Here's how the part is built. I have some questions about the finished solid (model axes, mm). A direction names the side the tool comes from. Give positions to 0.01 mm unless a question says otherwise; leave off trailing zeros. Write each loop counter-clockwise with the first axis right and the second up, starting at its lowest first coordinate (ties: lowest second). Pieces come first, ordered by that corner, then holes. Notation, with made-up numbers: (-22, 16.25) - (18, 16.25) arc R19 ccw to (18, 48.25) - close; hole circle Ø6 at (14.5, 57.25). An arc over 180 degrees is marked (long way). Write each question's results on one line, items separated by ' | '. Start each with the question number.
Item 1: Suppose I cut it at A-A on y = 18. Count the separate pieces of the cut face and the enclosed holes in it, then the cut area to 3 significant figures.
Item 2: Suppose I cut it at C-C on x = -25. List the corners of the cut face in (y, z) for me.
Item 3: Which directions (+Z, -Z, +X, -X, +Y, -Y) give clear straight access to the entire face, cutting with the end or side of a thin tool? Please do faces 1 (the flat face through (-50, -18, -18)), 2 (the flat face through (-39, -14, -28)), 3 (the flat face through (-3, 0, -16)).
Item 4: We'd pull the mould along Z, two halves only. Please class faces 4 (the flat face through (-28, 14, -26)), 5 (the flat face through (-1, 24, -1)), 6 (the cylindrical face through (-1.175, 2.494, -11.034)): +Z half, -Z half, draft (parallel to the pull), parting line (faces both ways), or undercut.
Item 5: Will these pins go through, and if not, where does the flat tip stop? P1, Ø3, axis at x = -55, y = 18, coming from the -Z side; P2, Ø5, axis at x = -79.5, y = -15.5, coming from the +Z side; P3, Ø2.5, axis at x = -43, y = -19, coming from the -Z side; P4, Ø4, axis at y = -18.5, z = -27, coming from the -X side.
Item 6: Suppose I cut it at B-B on y = 0. List the corners of the cut face in (x, z) for me.
Item 7: Suppose I cut it at D-D on z = -31. List the corners of the cut face in (x, y) for me, then the cut area to 3 significant figures.
Item 8: Please list where these lines run through material, in increasing order: line 1 along Y through (x, z) = (-24, -23.5); line 2 along Z through (x, y) = (-0.35, 0); line 3 along X through (y, z) = (-3, -6.5).
```python
from build123d import *

# Parameters (mm, degrees)
PAD_DEPTH         = 40
PAD001_DEPTH      = 25
POCKET_DEPTH      = 25.001
POCKET_DEPTH_BACK = -25.001
POCKET001_DEPTH   = 93
SKETCH003_R       = 1.7
POCKET002_DEPTH   = 40.001
SKETCH005_R       = 2.7
POCKET003_DEPTH   = 96.601
CHAMFER_SIZE      = 2
FILLET_R          = 1


with BuildPart() as part:
    # Sketch → Pad (new body)
    with BuildSketch(Plane.XY):
        Polygon((0, 25), (-96, 25), (-96, 11), (-3, 11), (-3, -11), (-96, -11), (-96, -25), (0, -25), align=None)
    extrude(amount=-PAD_DEPTH)

    # Sketch004 → Pad001 (join, symmetric)
    with BuildSketch(Plane.XZ):
        Polygon((0, -7), (0, -13), (0.6, -12.4), (0.6, -7.6), align=None)
        Polygon((0, -27), (0, -33), (0.6, -32.4), (0.6, -27.6), align=None)
    extrude(amount=PAD001_DEPTH, both=True)

    # Sketch001 → Pocket (cut, two sides)
    with BuildSketch(Plane.XZ) as pocket_sk:
        Polygon((-3, -40), (-96, -21), (-96, -18), (-3, -18), (-3, 0), (-97, 0), (-97, -40), align=None)
    extrude(amount=-POCKET_DEPTH, mode=Mode.SUBTRACT)
    extrude(pocket_sk.sketch, amount=-POCKET_DEPTH_BACK, mode=Mode.SUBTRACT)

    # Sketch002 → Pocket001 (cut)
    with BuildSketch(Plane.YZ.offset(-3)):
        Polygon((-22, -41), (-22, -21), (-14, -21), (-14, -40), (14, -40), (14, -21), (22, -21), (22, -41), align=None)
    extrude(amount=-POCKET001_DEPTH, mode=Mode.SUBTRACT)

    # Sketch003 → Pocket002 (cut, through all)
    with BuildSketch(Plane.XY):
        with Locations((-85, 18)):
            Circle(SKETCH003_R)
        with Locations((-25, 18)):
            Circle(SKETCH003_R)
        with Locations((-25, -18)):
            Circle(SKETCH003_R)
        with Locations((-85, -18)):
            Circle(SKETCH003_R)
        with Locations((-55, -18)):
            Circle(SKETCH003_R)
        with Locations((-55, 18)):
            Circle(SKETCH003_R)
    extrude(amount=-POCKET002_DEPTH, mode=Mode.SUBTRACT)

    # Sketch005 → Pocket003 (cut, through all)
    with BuildSketch(Plane.YZ.offset(0.6)):
        with Locations((0, -10)):
            Circle(SKETCH005_R)
        with Locations((0, -30)):
            Circle(SKETCH005_R)
    extrude(amount=-POCKET003_DEPTH, mode=Mode.SUBTRACT)

    # Chamfer
    chamfer_edges = [part.edges().sort_by_distance(p)[0] for p in [
        (-1.5, 25, 0),
        (-1.5, -25, 0),
    ]]
    chamfer(chamfer_edges, length=CHAMFER_SIZE)

    # Fillet
    fillet_edges = [part.edges().sort_by_distance(p)[0] for p in [
        (0, 0, 0),
        (0, 0, -40),
        (-3, 0, 0),
        (-3, 0, -40),
    ]]
    fillet(fillet_edges, radius=FILLET_R)


solid = part.part
```
Checked values:
1) separate pieces: 4 | enclosed holes: 0 | area: 374 mm^2
2) outline: (-25, -35.51) - (-22, -35.51) - (-22, -21) - (-19.7, -21) - (-19.7, -18) - (-25, -18) - close; (-16.3, -21) - (-14, -21) - (-14, -35.51) - (-11, -35.51) - (-11, -18) - (-16.3, -18) - close; (11, -35.51) - (14, -35.51) - (14, -21) - (16.3, -21) - (16.3, -18) - (11, -18) - close; (19.7, -21) - (22, -21) - (22, -35.51) - (25, -35.51) - (25, -18) - (19.7, -18) - close
3) face 1: +Z, -X, +Y, -Y | face 2: -Z, -X | face 3: +Z, -X
4) face 4: draft | face 5: +Z half | face 6: undercut
5) P1: passes through | P2: stops at z = -18 | P3: stops at z = -21 | P4: stops at x = -3
6) outline: (-3, -39) arc R1 ccw to (-2, -40) - (-1, -40) arc R1 ccw to (0, -39) - (0, -33) - (0.3, -32.7) - (-3, -32.7) - close; (-3, -27.3) - (0.3, -27.3) - (0, -27) - (0, -13) - (0.3, -12.7) - (-3, -12.7) - close; (-3, -7.3) - (0.3, -7.3) - (0, -7) - (0, -1) arc R1 ccw to (-1, 0) - (-2, 0) arc R1 ccw to (-3, -1) - close
7) outline: (-47.05, -25) - (0.6, -25) - (0.6, -2.51) - (-3, -2.51) - (-3, -11) - (-47.05, -11) - (-47.05, -14) - (-3, -14) - (-3, -22) - (-47.05, -22) - close; (-47.05, 11) - (-3, 11) - (-3, 2.51) - (0.6, 2.51) - (0.6, 25) - (-47.05, 25) - (-47.05, 22) - (-3, 22) - (-3, 14) - (-47.05, 14) - close | area: 691 mm^2
8) line 1: y = -25 to -22, -14 to -11, 11 to 14, 22 to 25 | line 2: z = -39.76 to -32.7, -27.3 to -12.7, -7.3 to -0.24 | line 3: x = -3 to 0
